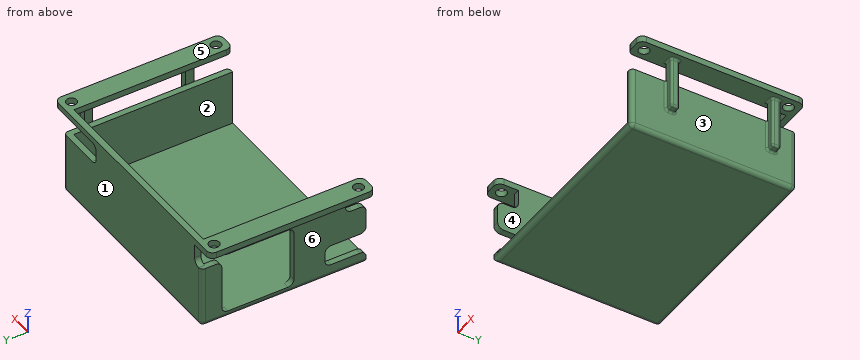
from build123d import *

# Parameters (mm, degrees)
SKETCH2_W           = 60
SKETCH2_H           = 40
SKETCH2_R           = 1.25
BOSS_EXTRUDE3_DEPTH = 1.5
SKETCH3_W           = 53
SKETCH3_H           = 40
BOSS_EXTRUDE4_DEPTH = 20
SKETCH7_W           = 50
SKETCH7_H           = 38.5
CUT_EXTRUDE4_DEPTH  = 20
SKETCH8_W           = 5
SKETCH8_H           = 40
CUT_EXTRUDE5_DEPTH  = 12.5
SKETCH11_W          = 5
SKETCH11_H          = 5
CUT_EXTRUDE8_DEPTH  = 2.5
SKETCH17_W          = 15
SKETCH17_H          = 17.5
SKETCH17_W_2        = 5
SKETCH17_H_2        = 10
CUT_EXTRUDE13_DEPTH = 2.5
SKETCH19_W          = 2
SKETCH19_H          = 2
BOSS_EXTRUDE5_DEPTH = 12.5
FILLET1_R           = 1.5
FILLET2_R           = 1.5
FILLET3_R           = 1
FILLET4_R           = 0.5
FILLET5_R           = 1.5


with BuildPart() as part:
    # Sketch2 → Boss-Extrude3 (new body)
    with BuildSketch(Plane.XY):
        with Locations((45.305986755, 42.83362131)):
            Rectangle(SKETCH2_W, SKETCH2_H)
        with Locations((17.805986755, 60.33362131)):
            Circle(SKETCH2_R, mode=Mode.SUBTRACT)
        with Locations((17.805986755, 25.33362131)):
            Circle(SKETCH2_R, mode=Mode.SUBTRACT)
        with Locations((72.805986755, 25.33362131)):
            Circle(SKETCH2_R, mode=Mode.SUBTRACT)
        with Locations((72.805986755, 60.33362131)):
            Circle(SKETCH2_R, mode=Mode.SUBTRACT)
    extrude(amount=BOSS_EXTRUDE3_DEPTH)

    # Sketch3 → Boss-Extrude4 (add)
    with BuildSketch(Plane(origin=(0, 0, 0), x_dir=(-1, 0, 0), z_dir=(0, 0, -1))):
        with Locations((-45.305986755, 42.83362131)):
            Rectangle(SKETCH3_W, SKETCH3_H)
    extrude(amount=BOSS_EXTRUDE4_DEPTH)

    # Sketch7 → Cut-Extrude4 (cut)
    with BuildSketch(Plane.XY.offset(1.5)):
        with Locations((45.305986755, 42.08362131)):
            Rectangle(SKETCH7_W, SKETCH7_H)
    extrude(amount=-CUT_EXTRUDE4_DEPTH, mode=Mode.SUBTRACT)

    # Sketch8 → Cut-Extrude5 (cut)
    with BuildSketch(Plane(origin=(71.805986755, 0, 0), x_dir=(0, 0, -1), z_dir=(1, 0, 0))):
        with Locations((2.5, 42.83362131)):
            Rectangle(SKETCH8_W, SKETCH8_H)
    extrude(amount=-CUT_EXTRUDE5_DEPTH, mode=Mode.SUBTRACT)

    # Sketch11 → Cut-Extrude8 (cut)
    with BuildSketch(Plane.ZY.offset(-18.805986755)):
        with Locations((-2.5, 60.33362131)):
            Rectangle(SKETCH11_W, SKETCH11_H)
        with Locations((-2.5, 25.33362131)):
            Rectangle(SKETCH11_W, SKETCH11_H)
    extrude(amount=-CUT_EXTRUDE8_DEPTH, mode=Mode.SUBTRACT)

    # Sketch17 → Cut-Extrude13 (cut)
    with BuildSketch(Plane.ZY.offset(-18.805986755)):
        with Locations((-11, 49.08362131)):
            Rectangle(SKETCH17_W, SKETCH17_H)
        with Locations((-14.5, 27.83362131)):
            Rectangle(SKETCH17_W_2, SKETCH17_H_2)
    extrude(amount=-CUT_EXTRUDE13_DEPTH, mode=Mode.SUBTRACT)

    # Sketch19 → Boss-Extrude5 (add)
    with BuildSketch(Plane(origin=(0, 0, 0), x_dir=(-1, 0, 0), z_dir=(0, 0, -1))):
        with Locations((-72.805986755, 32.33362131)):
            Rectangle(SKETCH19_W, SKETCH19_H)
        with Locations((-72.805986755, 56.83362131)):
            Rectangle(SKETCH19_W, SKETCH19_H)
    extrude(amount=BOSS_EXTRUDE5_DEPTH)

    # Fillet1
    fillet1_edges = [part.edges().sort_by_distance(p)[0] for p in [
        (70.305986755, 22.83362131, 0.75),
        (15.305986755, 62.83362131, 0.75),
        (75.305986755, 62.83362131, 0.75),
        (75.305986755, 22.83362131, 0.75),
        (15.305986755, 22.83362131, 0.75),
        (20.305986755, 22.83362131, 0.75),
    ]]
    fillet(fillet1_edges, radius=FILLET1_R)

    # Fillet2
    fillet2_edges = [part.edges().sort_by_distance(p)[0] for p in [
        (19.555986755, 57.83362131, -5),
        (19.555986755, 22.83362131, -5),
        (19.555986755, 27.83362131, -5),
        (19.555986755, 40.33362131, -18.5),
        (19.555986755, 40.33362131, -3.5),
        (19.555986755, 57.83362131, -3.5),
        (19.555986755, 57.83362131, -18.5),
        (19.555986755, 22.83362131, -17),
        (19.555986755, 32.83362131, -17),
        (19.555986755, 32.83362131, -12),
        (19.555986755, 22.83362131, -12),
        (59.305986755, 62.08362131, 0),
        (59.305986755, 62.08362131, -5),
    ]]
    fillet(fillet2_edges, radius=FILLET2_R)

    # Fillet3
    fillet3_edges = [part.edges().sort_by_distance(p)[0] for p in [
        (71.805986755, 62.83362131, -12.5),
        (71.805986755, 22.83362131, -12.5),
        (18.805986755, 62.83362131, -12.5),
        (71.805986755, 42.83362131, -20),
        (45.305986755, 22.83362131, -20),
        (18.805986755, 42.83362131, -20),
        (45.305986755, 62.83362131, -20),
    ]]
    fillet(fillet3_edges, radius=FILLET3_R)

    # Fillet4
    fillet4_edges = [part.edges().sort_by_distance(p)[0] for p in [
        (72.805986755, 55.83362131, 0),
        (72.805986755, 33.33362131, 0),
        (72.805986755, 31.33362131, 0),
        (73.805986755, 56.83362131, 0),
        (71.805986755, 32.33362131, 0),
        (73.805986755, 32.33362131, 0),
        (71.805986755, 56.83362131, 0),
        (72.805986755, 57.83362131, 0),
        (71.805986755, 32.33362131, -12.5),
        (71.805986755, 56.83362131, -12.5),
        (71.805986755, 33.33362131, -8.75),
        (71.805986755, 57.83362131, -8.75),
        (71.805986755, 55.83362131, -8.75),
        (73.805986755, 57.83362131, -6.25),
        (73.805986755, 33.33362131, -6.25),
        (71.805986755, 31.33362131, -8.75),
        (73.805986755, 31.33362131, -6.25),
        (73.805986755, 55.83362131, -6.25),
        (72.805986755, 55.83362131, -12.5),
        (73.805986755, 56.83362131, -12.5),
        (72.805986755, 57.83362131, -12.5),
        (72.805986755, 31.33362131, -12.5),
        (73.805986755, 32.33362131, -12.5),
        (72.805986755, 33.33362131, -12.5),
    ]]
    fillet(fillet4_edges, radius=FILLET4_R)

    # Fillet5
    # the kernel refuses this fillet: 1.5 mm, written as the material it adds along each edge
    with BuildSketch(Plane(origin=(21.305986755, 62.83362131, -5), x_dir=(-1, 0, 0), z_dir=(0, -1, 0))) as fillet5_piece_1:
        with BuildLine():
            CenterArc((FILLET5_R, -FILLET5_R), FILLET5_R, 90, 90)
            Line((0, -FILLET5_R), (0, 0))
            Line((0, 0), (FILLET5_R, 0))
        make_face()
    extrude(amount=1.5)


solid = part.part
Verification items for the finished model (mm, model axes). Face numbers are marked on the shaded views. A direction names the side the tool comes from. Coordinates: 2 decimals unless noted, no trailing zeros. Order: outer loops, then holes, each group sorted by start corner. A loop starts at its lowest first (then second) coordinate and runs counter-clockwise, first axis right, second up. Notation, with made-up numbers: M -33.5,-12 L -28.5,-12 A14 ccw -28.5,-8 Z; hole C 11,15 d3. An arc over 180 degrees is marked long. One line per item, written item: value. Start each with the question number.
Item 1: Gauge pin test, flat ends, axial feed: pin 1 (0.8 mm diameter, centred on x = 73, y = 32.5, fed in from -Z); pin 2 (12 mm diameter, centred on y = 31.5, z = -17.5, fed in from -X); pin 3 (1.5 mm diameter, centred on x = 50.5, y = 34, fed in from +Z). Record the tip position at first contact, or that the pin passes through.
Item 2: Sectioned sample at B-B (y = 30). Enter the section's corners in (x, z), then the cut area to 3 significant figures.
Item 3: Mould release check, pull along X, two halves, no side actions. Record for the marked faces 4, 5 and 6: released by +X, released by -X, zero draft, split by the parting line, or undercut.
Item 4: Sectioned sample at C-C (y = 36). Enter the section's corners in (x, z), then the cut area to 3 significant figures.
Item 5: Scan lines: probe 1 along X at (y, z) = (49, 0.25); probe 2 along X at (y, z) = (35, -15.5); probe 3 along Y at (x, z) = (73, -1.25). Record each from-to range of solid material in increasing order.
Item 6: Sectioned sample at D-D (z = -14.5). Enter the section's corners in (x, y).
Item 7: Access from +Z, -Z, +X, -X, +Y, -Y to the whole of each face (thin tool, end or side, straight path). Record for the marked faces 1, 2 and 3.
Item 8: Sectioned sample at A-A (x = 64). Enter the section's corners in (y, z), then the cut area to 3 significant figures.
Conclusion:
1. pin 1: stops at z = -12.5
1. pin 2: stops at x = 18.81
1. pin 3: stops at z = -18.5
2. outline: M 15.31,0 L 18.81,0 L 18.81,-12 L 20.31,-12 L 20.31,1.5 L 15.31,1.5 Z; M 18.81,-19 A1 ccw 19.81,-20 L 70.81,-20 A1 ccw 71.81,-19 L 71.81,-5 L 70.31,-5 L 70.31,-18.5 L 20.31,-18.5 L 20.31,-17 L 18.81,-17 Z; M 70.31,0 L 75.31,0 L 75.31,1.5 L 70.31,1.5 Z
2. area: 135 mm^2
3. face 4: undercut
3. face 5: zero draft
3. face 6: released by -X
4. outline: M 15.31,0 L 18.81,0 L 18.81,-19 A1 ccw 19.81,-20 L 70.81,-20 A1 ccw 71.81,-19 L 71.81,-5 L 70.31,-5 L 70.31,-18.5 L 20.31,-18.5 L 20.31,1.5 L 15.31,1.5 Z; M 70.31,0 L 75.31,0 L 75.31,1.5 L 70.31,1.5 Z
4. area: 142 mm^2
5. probe 1: x = 15.31 to 20.31, 70.31 to 75.31
5. probe 2: x = 18.81 to 20.31, 70.31 to 71.81
5. probe 3: y = 31.33 to 33.33, 55.83 to 57.83
6. outline: M 18.81,32.83 L 20.31,32.83 L 20.31,40.33 L 18.81,40.33 Z; M 18.81,57.83 L 20.31,57.83 L 20.31,61.33 L 70.31,61.33 L 70.31,22.83 L 70.81,22.83 A1 ccw 71.81,23.83 L 71.81,61.83 A1 ccw 70.81,62.83 L 19.81,62.83 A1 ccw 18.81,61.83 Z
7. face 1: +Z, -Z, +X, -X, +Y
7. face 2: +Z, -Y
7. face 3: -Z, +X
8. outline: M 22.83,-19 A1 ccw 23.83,-20 L 61.83,-20 A1 ccw 62.83,-19 L 62.83,-5 L 61.33,-5 L 61.33,-18.5 L 22.83,-18.5 Z; M 61.33,0 L 62.83,0 L 62.83,1.5 L 61.33,1.5 Z
8. area: 82.1 mm^2
